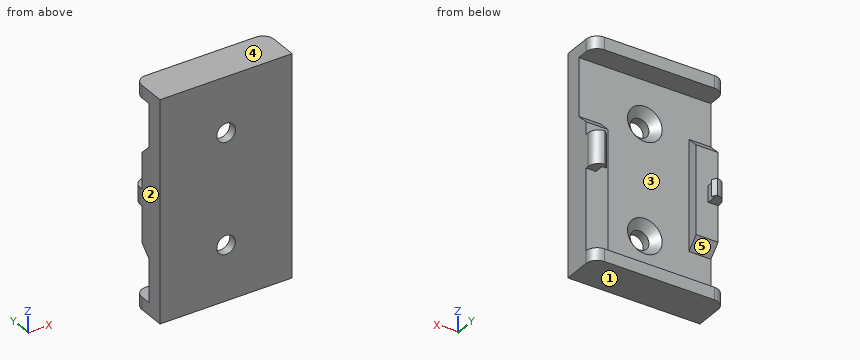
Autodesk Inventor part; units mm, degrees
ref_plane "YZ Plane" through (0, 0, 0) normal (1, 0, 0) x (0, 1, 0)
ref_plane "XZ Plane" through (0, 0, 0) normal (0, 1, 0) x (-1, 0, 0)
ref_plane "XY Plane" through (0, 0, 0) normal (0, 0, 1) x (1, 0, 0)
sketch "Skizze1" plane through (0, 0, 0) normal (0, 1, 0) x (-1, 0, 0)
  line L0 (0, 0) -> (24, 0)
  line L1 (24, 0) -> (24, -40)
  line L2 (24, -40) -> (0, -40)
  line L3 (0, -40) -> (0, 0)
  dimension "d0" = 40
  dimension "d1" = 24
extrude "Extrusion1" add sketch "Skizze1" along normal blind 3
sketch "Skizze2" plane through (0, 3, 0) normal (0, 1, 0) x (1, 0, 0)
  line L0 (-24, 40) -> (-24, 0)
  line L1 (0, 0) -> (0, 40)
  line L2 (-24, 0) -> (0, 0)
  line L3 (0, 0) -> (0, 2.25)
  line L4 (0, 2.25) -> (-24, 2.25)
  line L5 (-24, 2.25) -> (-24, 0)
  line L6 (0, 40) -> (-24, 40)
  line L7 (-24, 40) -> (0, 40)
  line L8 (0, 40) -> (0, 37.75)
  line L9 (0, 37.75) -> (-24, 37.75)
  line L10 (-24, 37.75) -> (-24, 40)
  dimension "d4" = 2.25
  dimension "d5" = 2.25
extrude "Extrusion2" add sketch "Skizze2" along normal blind 4 contours L6 L1 L9 L0 | L4 L1 L2 L0
sketch "Skizze4" plane through (0, 3, 0) normal (0, 1, 0) x (1, 0, 0)
  line L0 (0, 2.25) -> (-24, 2.25)
  line L1 (0, 2.25) -> (-1.8184, 2.25)
  line L2 (0, 37.75) -> (-1.8184, 37.75)
  line L3 (-24.0183, 2.25) -> (-21.7244, 2.25)
  line L4 (-24, 37.75) -> (-21.1801, 37.75)
  line L5 (0, 37.75) -> (-4, 37.75)
  line L6 (-4, 37.75) -> (-4, 12.75)
  line L7 (-4, 12.75) -> (0, 12.75)
  line L8 (0, 12.75) -> (0, 37.75)
  line L9 (-24, 37.75) -> (-24, 2.25)
  line L10 (-24, 10) -> (-20, 10)
  line L11 (-20, 10) -> (-20, 30)
  line L12 (-20, 30) -> (-24, 30)
  line L13 (-24, 30) -> (-24, 10)
  line L14 (-24, 0) -> (0, 0)
  dimension "d25" = 25
  dimension "d26" = 4
  dimension "d27" = 4
  dimension "d29" = 20
  dimension "d30" = 10
extrude "Extrusion4" add sketch "Skizze4" along normal blind 2
sketch "Skizze5" plane through (0, 5, 0) normal (0, 1, 0) x (1, 0, 0)
  line L0 (-24, 30) -> (-24, 10)
  line L1 (-24, 20) -> (0, 20)
  line L2 (0, 0) -> (0, 40)
  line L3 (-24, 18.5) -> (-22.2, 18.5)
  line L4 (-22.2, 18.5) -> (-22.2, 21.5)
  line L5 (-22.2, 21.5) -> (-24, 21.5)
  line L6 (-24, 21.5) -> (-24, 18.5)
  line L7 (0, 17) -> (-1.8, 17)
  line L8 (-1.8, 17) -> (-1.8, 23)
  line L9 (-1.8, 23) -> (0, 23)
  line L10 (0, 23) -> (0, 17)
  point P0 (-23.1, 18.5)
  point P1 (0, 23)
  dimension "d33" = 3
  dimension "d34" = 1.8
  dimension "d35" = 1.8
  dimension "d36" = 6
extrude "Extrusion5" add sketch "Skizze5" along normal blind 2.5
sketch "Skizze6" plane through (-1.8, 5, -23) normal (-1, 0, 0) x (0, 0, 1)
  line L0 (0, 0) -> (0, 2.5)
  line L1 (6, 0) -> (6, 2.5)
  line L2 (0, 2.5) -> (6, 2.5)
  line L3 (6, 2.5) -> (6, 1.7)
  line L4 (6, 1.7) -> (0, 1.7)
  line L5 (0, 1.7) -> (0, 2.5)
  point P0 (23, -5)
  point P1 (0, 1.7)
  dimension "d39" = 0.8
extrude "Extrusion6" add sketch "Skizze6" along normal blind 1
sketch "Skizze7" plane through (0, 5, -23) normal (0, 0, -1) x (-1, 0, 0)
  line L0 (2.8, 2.5) -> (2.8, 1.7)
  line L1 (2.8, 1.5) -> (1.8, 2.5)
  line L2 (0, 2.5) -> (2.8, 2.5)
  line L3 (1.8, 2.5) -> (2.8, 2.5)
  line L4 (2.8, 2.5) -> (2.8, 1.5)
  point P0 (0, -5)
  dimension "d42" = 1
  dimension "d43" = 1
extrude "Extrusion7" cut sketch "Skizze7" against normal blind 10
sketch "Skizze9" plane through (-22.2, 5, -18.5) normal (1, 0, 0) x (0, 0, -1)
  line L0 (0, 0) -> (0, 2.5)
  line L1 (3, 0) -> (3, 2.5)
  line L2 (0, 2.5) -> (3, 2.5)
  line L3 (3, 2.5) -> (3, 1.7)
  line L4 (3, 1.7) -> (0, 1.7)
  line L5 (0, 1.7) -> (0, 2.5)
  line L6 (3, 0) -> (0, 0)
  point P0 (-18.5, -5)
  point P1 (0, 1.7)
  dimension "d46" = 1.7
extrude "Extrusion8" add sketch "Skizze9" along normal blind 0.5 contours L0 L2 L1 L4
sketch "Skizze11" plane through (-22.2, 5, -21.5) normal (0, 0, -1) x (-1, 0, 0)
  line L0 (-0.5, 2.5) -> (-0.5, 1.7)
  line L1 (-0.5, 1.7) -> (0, 2.5)
  line L2 (1.8, 2.5) -> (-0.5, 2.5)
  line L3 (-0.5, 1.7) -> (-0.5, 2.5)
  line L4 (-0.5, 2.5) -> (0, 2.5)
  point P0 (-22.2, -5)
  dimension "d49" = 0.5
extrude "Extrusion9" cut sketch "Skizze11" against normal blind 10
chamfer "Fasen1" distance 2 angle 45 3 edges at (-22, 5, -30) (-22, 5, -10) (-2, 5, -12.75)
fillet "Rundung1" radius 2 6 edges at (0, 7.5, -20) (-24, 7.5, -20) (-24, 7, -1.125) (0, 7, -1.125) (-24, 7, -38.875) (0, 7, -38.875)
sketch "Skizze12" plane through (0, 3, 0) normal (0, 1, 0) x (1, 0, 0)
  line L0 (-24, 0) -> (0, 0)
  line L1 (-12, 0) -> (-12, 40)
  line L2 (0, 40) -> (-24, 40)
  circle A0 centre (-12, 10) radius 2
  circle A1 centre (-12, 30) radius 2
  line L3 (-24, 40) -> (-24, 0)
  line L4 (-24, 20) -> (0, 20) construction
  line L5 (0, 17) -> (0, 23)
  dimension "d56" = 4
  dimension "d57" = 4
  dimension "d58" = 20
hole "Bohrung1" at (-12, 3, -10) at (-12, 3, -30) direction (0, -1, 0) diameter 3.4 depth 8.8 tip angle 118 countersink diameter 6.3 countersink angle 90
properties part number "Halter_Treiber_LED_2"
Here's how the part is built. I have some questions about the finished solid (model axes, mm). Face numbers are marked on the shaded views. A direction names the side the tool comes from. Coordinates: 2 decimals unless noted, no trailing zeros. Order: outer loops, then holes, each group sorted by start corner. A loop starts at its lowest first (then second) coordinate and runs counter-clockwise, first axis right, second up. Notation, with made-up numbers: M 24.5,84.25 L 30.5,84.25 A30 ccw 30.5,115.25 Z; hole C 63,10.5 d8. An arc over 180 degrees is marked long. Answer as a JSON object with one key per item and string values. Group by question number.
(1) Which directions (+Z, -Z, +X, -X, +Y, -Y) give clear straight access to the entire face, cutting with the end or side of a thin tool? Please do the marked faces 4 and 5.
(2) Suppose I cut it at B-B, the plane y = 0.5. Please give me the cut outline in (x, z).
(3) Suppose I cut it at A-A, the plane x = -12. Please give me the cut outline in (y, z), then the cut area to 3 significant figures.
(4) Suppose I cut it at C-C, the plane y = 4.5. Please give me the cut outline in (x, z).
(5) Suppose I cut it at D-D, the plane x = -17.75. Please give me the cut outline in (y, z).
(6) If we mould it in two halves opening along Z, with no side actions, what happens to the marked faces 1, 2 and 3? For each: released by +Z, released by -Z, zero draft, split by the parting line, or undercut.
(7) For pin 1 (2 mm diameter, centred on x = -8, z = -11, fed in from +Y); pin 2 (8 mm diameter, centred on x = -5, z = -27, fed in from +Y); pin 3 (1.1 mm diameter, centred on x = -14.5, z = -1.5, fed in from +Y), each with a flat end and sliding along its axis, tell me the tip position at first contact or that it passes through.
(8) I need wall thicknesses on probe 1 along Z at (x, y) = (-12, 1.25); probe 2 along X at (y, z) = (0.75, -10); probe 3 along Z at (x, y) = (-18.5, 6.5). Which ranges of each line are inside material? Lowest first, please.
Values found:
{
 "1": {"face 4": "+Z, +X, -X, +Y, -Y", "face 5": "-X, +Y"},
 "2": {"outline": "M -24,-40 L 0,-40 L 0,0 L -24,0 Z; hole C -12,-30 d3.4; hole C -12,-10 d3.4"},
 "3": {"outline": "M 0,-40 L 7,-40 L 7,-37.75 L 3,-37.75 L 3,-33.15 L 1.55,-31.7 L 0,-31.7 Z; M 0,-28.3 L 1.55,-28.3 L 3,-26.85 L 3,-13.15 L 1.55,-11.7 L 0,-11.7 Z; M 0,-8.3 L 1.55,-8.3 L 3,-6.85 L 3,-2.25 L 7,-2.25 L 7,0 L 0,0 Z", "area": "113 mm^2"},
 "4": {"outline": "M -24,-40 L 0,-40 L 0,-14.25 L -4,-14.25 L -4,-37.75 L -24,-37.75 Z; M -24,-28.5 L -20,-28.5 L -20,-11.5 L -24,-11.5 Z; M -24,-2.25 L 0,-2.25 L 0,0 L -24,0 Z"},
 "5": {"outline": "M 0,-40 L 7,-40 L 7,-37.75 L 3,-37.75 L 3,-2.25 L 7,-2.25 L 7,0 L 0,0 Z"},
 "6": {"face 1": "released by -Z", "face 2": "zero draft", "face 3": "undercut"},
 "7": {"pin 1": "stops at y = 3", "pin 2": "stops at y = 5", "pin 3": "stops at y = 7"},
 "8": {"probe 1": "z = -40 to -31.7, -28.3 to -11.7, -8.3 to 0", "probe 2": "x = -24 to -13.7, -10.3 to 0", "probe 3": "z = -40 to -37.75, -2.25 to 0"}
}
